```python
from build123d import *

# Parameters (mm, degrees)
SKETCH1_W           = 100
SKETCH1_H           = 64
BOSS_EXTRUDE1_DEPTH = 6
SKETCH2_R           = 9
SKETCH2_R_2         = 3.5
CUT_EXTRUDE1_DEPTH  = 10
LPATTERN1_COUNT     = 2
LPATTERN1_PITCH     = 60
BOSS_EXTRUDE2_DEPTH = 10
SKETCH4_W           = 6
SKETCH4_H           = 6
BOSS_EXTRUDE3_DEPTH = 20
SKETCH5_W           = 97
SKETCH5_H           = 16
BOSS_EXTRUDE4_DEPTH = 3
LPATTERN4_COUNT     = 2
LPATTERN4_PITCH     = 67
SKETCH6_W           = 16
SKETCH6_H           = 70
BOSS_EXTRUDE5_DEPTH = 3
SKETCH7_W           = 5.405235292
SKETCH7_H           = 22
CUT_EXTRUDE2_DEPTH  = 6
SKETCH8_W           = 6
SKETCH8_H           = 62
BOSS_EXTRUDE6_DEPTH = 10
SKETCH9_R           = 2.5
CUT_EXTRUDE3_DEPTH  = 10
LPATTERN5_COUNT     = 2
LPATTERN5_PITCH     = 15
FILLET1_R           = 2
SKETCH10_R          = 2.5
CUT_EXTRUDE4_DEPTH  = 10
LPATTERN6_COUNT     = 2
LPATTERN6_PITCH     = 30


with BuildPart() as part:
    # Sketch1 → Boss-Extrude1 (new body)
    with BuildSketch(Plane.XY):
        with Locations((-4.657534247, -15.767123288)):
            Rectangle(SKETCH1_W, SKETCH1_H)
    extrude(amount=BOSS_EXTRUDE1_DEPTH)

    # Sketch2 → Cut-Extrude1 (cut)
    with BuildSketch(Plane.XY.offset(6)):
        with Locations((-35.657534247, -15.767123288)):
            Circle(SKETCH2_R)
        with Locations((-35.657534247, 8.232876712)):
            Circle(SKETCH2_R_2)
        with Locations((-35.657534247, -39.767123288)):
            Circle(SKETCH2_R_2)
    cut_extrude1 = extrude(amount=-CUT_EXTRUDE1_DEPTH, mode=Mode.SUBTRACT)

    # LPattern1: Cut-Extrude1 ×2
    with Locations(*[(i * LPATTERN1_PITCH, 0, 0) for i in range(1, LPATTERN1_COUNT)]):
        add(cut_extrude1, mode=Mode.SUBTRACT)

    # Sketch3 → Boss-Extrude2 (add)
    with BuildSketch(Plane(origin=(0, 0, 0), x_dir=(-1, 0, 0), z_dir=(0, 0, -1))):
        Polygon((48.657534247, -47.767123288), (48.657534247, 16.232876712), (51.657534247, 16.232876712), (51.657534247, -47.767123288), (51.657534247, -67.767123288), (48.657534247, -67.767123288), align=None)
    extrude(amount=BOSS_EXTRUDE2_DEPTH)

    # Sketch4 → Boss-Extrude3 (add)
    with BuildSketch(Plane(origin=(0, -47.767123288, 0), x_dir=(-1, 0, 0), z_dir=(0, -1, 0))):
        with Locations((51.657534247, -3)):
            Rectangle(SKETCH4_W, SKETCH4_H)
    extrude(amount=BOSS_EXTRUDE3_DEPTH)

    # Sketch5 → Boss-Extrude4 (add)
    with BuildSketch(Plane(origin=(0, -47.767123288, 0), x_dir=(-1, 0, 0), z_dir=(0, -1, 0))):
        with Locations((3.157534247, 2)):
            Rectangle(SKETCH5_W, SKETCH5_H)
    boss_extrude4 = extrude(amount=BOSS_EXTRUDE4_DEPTH)

    # LPattern4: Boss-Extrude4 ×2
    with Locations(*[(0, i * LPATTERN4_PITCH, 0) for i in range(1, LPATTERN4_COUNT)]):
        add(boss_extrude4)

    # Sketch6 → Boss-Extrude5 (add)
    with BuildSketch(Plane(origin=(45.342465753, 0, 0), x_dir=(0, 0, -1), z_dir=(1, 0, 0))):
        with Locations((2, -15.767123288)):
            Rectangle(SKETCH6_W, SKETCH6_H)
    extrude(amount=BOSS_EXTRUDE5_DEPTH)

    # Sketch7 → Cut-Extrude2 (cut)
    with BuildSketch(Plane(origin=(0, 0, 0), x_dir=(-1, 0, 0), z_dir=(0, 0, -1))):
        with Locations((54.360151893, 5.232876712)):
            Rectangle(SKETCH7_W, SKETCH7_H)
    extrude(amount=-CUT_EXTRUDE2_DEPTH, mode=Mode.SUBTRACT)

    # Sketch8 → Boss-Extrude6 (add)
    with BuildSketch(Plane.ZY.offset(54.657534247)):
        with Locations((3, -36.767123288)):
            Rectangle(SKETCH8_W, SKETCH8_H)
    extrude(amount=BOSS_EXTRUDE6_DEPTH)

    # Sketch9 → Cut-Extrude3 (cut)
    with BuildSketch(Plane(origin=(0, 0, 0), x_dir=(-1, 0, 0), z_dir=(0, 0, -1))):
        with Locations((58.657534247, -57.767123288)):
            Circle(SKETCH9_R)
    cut_extrude3 = extrude(amount=-CUT_EXTRUDE3_DEPTH, mode=Mode.SUBTRACT)

    # LPattern5: Cut-Extrude3 ×2
    with Locations(*[(0, i * LPATTERN5_PITCH, 0) for i in range(1, LPATTERN5_COUNT)]):
        add(cut_extrude3, mode=Mode.SUBTRACT)

    # Fillet1
    fillet1_edges = [part.edges().sort_by_distance(p)[0] for p in [
        (-51.657534247, 19.232876712, -2),
        (48.342465753, -50.767123288, -2),
        (48.342465753, 19.232876712, -2),
        (-48.657534247, -50.767123288, -2),
    ]]
    fillet(fillet1_edges, radius=FILLET1_R)

    # Sketch10 → Cut-Extrude4 (cut)
    with BuildSketch(Plane(origin=(48.342465753, 0, 0), x_dir=(0, 0, -1), z_dir=(1, 0, 0))):
        with Locations((4, -0.767123288)):
            Circle(SKETCH10_R)
    cut_extrude4 = extrude(amount=-CUT_EXTRUDE4_DEPTH, mode=Mode.SUBTRACT)

    # LPattern6: Cut-Extrude4 ×2
    with Locations(*[(0, -i * LPATTERN6_PITCH, 0) for i in range(1, LPATTERN6_COUNT)]):
        add(cut_extrude4, mode=Mode.SUBTRACT)


solid = part.part
```
Design review of the part built by this model. Coordinates are the model's own, in mm. A direction names the side the tool comes from. Coordinates: 2 decimals unless noted, no trailing zeros. Write each loop counter-clockwise with the first axis right and the second up, starting at its lowest first coordinate (ties: lowest second). Pieces come first, ordered by that corner, then holes. Notation, with made-up numbers: M -4.5,25.25 L 14.5,25.25 A10 cw 14.5,36.25 Z; hole C 79,-9 d9. An arc over 180 degrees is marked long. Answer as a JSON object with one key per item and string values.
Item 1: Draft analysis for pull direction Z (two halves, no side actions). For faces 5 (the flat face through (-7, -15, 6)), 6 (the cylindrical face through (46.863, -0.016, -6.385)), 7 (the flat face through (-48.658, -60, -2)), state which applies: pulls with the +Z half, pulls with the -Z half, needs draft (parallel to the pull), parting line crosses it, or undercut.
Outcome:
{"face 5": "pulls with the +Z half", "face 6": "undercut", "face 7": "needs draft"}
Item 2: Add section C-C, the plane y = 9.5. Give the boundary of the cut face in (x, z).
Outcome:
{"outline": "M -51.66,-10 L -48.66,-10 L -48.66,0 L -38.92,0 L -38.92,6 L -51.66,6 Z; M -32.39,0 L 21.08,0 L 21.08,6 L -32.39,6 Z; M 27.61,0 L 45.34,0 L 45.34,-10 L 48.34,-10 L 48.34,6 L 27.61,6 Z"}
Item 3: Insertion check: pin 1 Ø5 at (x, y) = (25, -36.5) entering from +Z; pin 2 Ø8 at (x, y) = (-11, -30.5) entering from -Z; pin 3 Ø1 at (x, z) = (-2, -7.5) entering from -Y; pin 4 Ø4.5 at (y, z) = (-0.77, -4) entering from +X. Each pin has a flat end and moves straight along its axis. Give the tip position at first contact, or say it passes through.
Outcome:
{"pin 1": "z = 6", "pin 2": "z = 0", "pin 3": "y = -50.77", "pin 4": "x = -48.66"}
Item 4: Wall thickness on probe 1 along Y at (x, z) = (-35.5, 4); probe 2 along X at (y, z) = (-22, -4.5); probe 3 along Y at (x, z) = (-2.5, -1.75): over which ranges is each line inside the solid? List them lowest first.
Outcome:
{"probe 1": "-50.77 to -43.26, -36.27 to -24.77, -6.77 to 4.74, 11.73 to 19.23", "probe 2": "-51.66 to -48.66, 45.34 to 48.34", "probe 3": "-50.77 to -47.77, 16.23 to 19.23"}
Item 5: Machinability: for faces 1 (the flat face through (-58, -37, 0)), 2 (the flat face through (-1, -50.767, -2)), 3 (the flat face through (-1, -47.767, -5)), 4 (the cylindrical face through (46.86, -28.29, -3.67)), which of the approach directions +Z, -Z, +X, -X, +Y, -Y give a long, thin tool a straight path to every point of the face, cutting with its end or side? Answer none if there is none.
Outcome:
{"face 1": "-Z, -X, +Y, -Y", "face 2": "+Z, -Z, +X, -Y", "face 3": "-Z", "face 4": "+X"}
Item 6: Add section D-D, the plane y = -38. Give the boundary of the cut face in (x, z), and give its area (3 significant figures).
Outcome:
{"outline": "M -64.66,0 L -51.66,0 L -51.66,-10 L -48.66,-10 L -48.66,0 L -38.68,0 L -38.68,6 L -64.66,6 Z; M -32.64,0 L 21.32,0 L 21.32,6 L -32.64,6 Z; M 27.36,0 L 45.34,0 L 45.34,-10 L 48.34,-10 L 48.34,6 L 27.36,6 Z", "area": "665 mm²"}
Item 7: Add section B-B, the plane y = -13. Give the boundary of the cut face in (x, z), and give its area (3 significant figures).
Outcome:
{"outline": "M -64.66,0 L -51.66,0 L -51.66,-10 L -48.66,-10 L -48.66,0 L -44.22,0 L -44.22,6 L -64.66,6 Z; M -27.09,0 L 15.78,0 L 15.78,6 L -27.09,6 Z; M 32.91,0 L 45.34,0 L 45.34,-10 L 48.34,-10 L 48.34,6 L 32.91,6 Z", "area": "532 mm²"}
Item 8: Add section A-A, the plane z = -4. Give the boundary of the cut face in (x, y), and give its area (3 significant figures).
Outcome:
{"outline": "M -51.66,-67.77 L -48.66,-67.77 L -48.66,-52.77 A2 cw -46.66,-50.77 L 46.34,-50.77 A2 ccw 48.34,-48.77 L 48.34,-33.27 L 45.34,-33.27 L 45.34,-47.77 L -48.66,-47.77 L -48.66,16.23 L 45.34,16.23 L 45.34,1.73 L 48.34,1.73 L 48.34,17.23 A2 ccw 46.34,19.23 L -49.66,19.23 A2 ccw -51.66,17.23 Z; M 45.34,-28.27 L 48.34,-28.27 L 48.34,-3.27 L 45.34,-3.27 Z", "area": "1,000 mm²"}
